from build123d import *

# Parameters (mm, degrees)
SKETCH1_W           = 200
SKETCH1_H           = 180
BOSS_EXTRUDE1_DEPTH = 3
SKETCH2_W           = 200
SKETCH2_H           = 140
BOSS_EXTRUDE2_DEPTH = 5
SKETCH6_W           = 200
SKETCH6_H           = 179.869705491
BOSS_EXTRUDE3_DEPTH = 24
SKETCH7_W           = 155
SKETCH7_H           = 24
CUT_EXTRUDE1_DEPTH  = 179.869705491
SKETCH8_R           = 2
BOSS_EXTRUDE4_DEPTH = 155
SKETCH9_W           = 155
SKETCH9_H           = 5
BOSS_EXTRUDE5_DEPTH = 10
CUT_EXTRUDE3_DEPTH  = 174.869705491
SKETCH12_R          = 7.1
CUT_EXTRUDE4_DEPTH  = 2


with BuildPart() as part:
    # Sketch1 → Boss-Extrude1 (new body)
    with BuildSketch(Plane(origin=(0, 0, 0), x_dir=(1, 0, 0), z_dir=(0, 1, 0))):
        Rectangle(SKETCH1_W, SKETCH1_H)
    extrude(amount=BOSS_EXTRUDE1_DEPTH)

    # Sketch2 → Boss-Extrude2 (add)
    with BuildSketch(Plane.XZ):
        with Locations((0, 20)):
            Rectangle(SKETCH2_W, SKETCH2_H)
    extrude(amount=BOSS_EXTRUDE2_DEPTH)

    # Sketch6 → Boss-Extrude3 (add)
    with BuildSketch(Plane(origin=(0, 3, 0), x_dir=(1, 0, 0), z_dir=(0, 1, 0))):
        with Locations((0, -0.065147254)):
            Rectangle(SKETCH6_W, SKETCH6_H)
    extrude(amount=BOSS_EXTRUDE3_DEPTH)

    # Sketch7 → Cut-Extrude1 (cut)
    with BuildSketch(Plane(origin=(0, 0, -89.869705491), x_dir=(-1, 0, 0), z_dir=(0, 0, -1))):
        with Locations((-17.5, 15)):
            Rectangle(SKETCH7_W, SKETCH7_H)
    extrude(amount=-CUT_EXTRUDE1_DEPTH, mode=Mode.SUBTRACT)

    # Sketch8 → Boss-Extrude4 (add)
    with BuildSketch(Plane.ZY.offset(-95)):
        with Locations(Location((-79.869705491, 13.5, 0), (0, 0, 180))):
            Circle(SKETCH8_R)
    extrude(amount=BOSS_EXTRUDE4_DEPTH)

    # Sketch9 → Boss-Extrude5 (add)
    with BuildSketch(Plane(origin=(0, 3, 0), x_dir=(1, 0, 0), z_dir=(0, 1, 0))):
        with Locations((17.5, -87.5)):
            Rectangle(SKETCH9_W, SKETCH9_H)
    extrude(amount=BOSS_EXTRUDE5_DEPTH)

    # Sketch11 → Cut-Extrude3 (cut)
    with BuildSketch(Plane(origin=(0, 0, -89.869705491), x_dir=(-1, 0, 0), z_dir=(0, 0, -1))):
        Polygon((60, 3), (98, 3), (98, 25), (62, 25), (62, 7), (60, 7), align=None)
    extrude(amount=-CUT_EXTRUDE3_DEPTH, mode=Mode.SUBTRACT)

    # Sketch12 → Cut-Extrude4 (cut)
    with BuildSketch(Plane(origin=(0, 27, 0), x_dir=(1, 0, 0), z_dir=(0, 1, 0))):
        with Locations(Location((-70, -45.032573627, 0), (0, 0, 270))):
            Circle(SKETCH12_R)
        with Locations(Location((-70, -67.516286814, 0), (0, 0, 270))):
            Circle(SKETCH12_R)
        with Locations(Location((-90, -67.516286814, 0), (0, 0, 180))):
            Circle(SKETCH12_R)
        with Locations(Location((-90, -45.032573627, 0), (0, 0, 180))):
            Circle(SKETCH12_R)
    extrude(amount=-CUT_EXTRUDE4_DEPTH, mode=Mode.SUBTRACT)


solid = part.part
Input: part model. Units: mm. Frame: model coordinates. A direction names the side the tool comes from. Give positions to 0.01 mm unless a question says otherwise; leave off trailing zeros. Order: outer loops, then holes, each group sorted by start corner. A loop starts at its lowest first (then second) coordinate and runs counter-clockwise, first axis right, second up. Notation, with made-up numbers: (62.25, 84) - (83.25, 84) arc R25 cw to (83.25, 107) - close; hole circle Ø9 at (-3.75, 50). An arc over 180 degrees is marked (long way). Answer as a JSON object with one key per item and string values. Group by question number.
Q1. First-contact query: pin 1 Ø13 at (x, z) = (-70, 67.52) entering from +Y; pin 2 Ø10 at (x, y) = (67, 13) entering from -Z; pin 3 Ø4 at (x, y) = (-38.5, -2.5) entering from -Z. Flat tips, straight axial feed; report the tip coordinate or a pass-through.
Q2. Cut plane A-A, the plane y = 19. Output: boundary loops of the cut face in (x, z).
Q3. Line query: probe 1 along X at (y, z) = (21, -41.5); probe 2 along Z at (x, y) = (-90, 25.45); probe 3 along Y at (x, z) = (39.5, -46.5). Output: solid intervals per line, ascending.
Q4. Set-up query: faces 5 (the face through (-1, 3, -4)), 6 (the face through (-82.907, 26.014, 67.828)), 7 (the face through (16, 13, 87)). Return all of +Z, -Z, +X, -X, +Y, -Y with unobstructed straight access to the full face (end or side cutting, diameter ignored); none if empty.
Q5. Mould query, pull axis Z, two halves, no side actions, for faces 1 (the face through (-80, 25, -4)), 2 (the face through (-24, 7, 90)), 3 (the face through (-1, -2, -50)), 4 (the face through (-72.7, 26, 51.6)). Classes: pulls with the +Z half, pulls with the -Z half, needs draft (parallel to the pull), parting line crosses it, or undercut.
Q6. Cut plane C-C, the plane x = -70. Output: boundary loops of the cut face in (y, z), then the cut area to 3 significant figures.
Q7. Cut plane B-B, the plane x = 33. Output: boundary loops of the cut face in (y, z), then the cut area to 3 significant figures.
Q8. Cut plane D-D, the plane z = 3.5. Output: boundary loops of the cut face in (x, y).
Results:
{
 "1": {"pin 1": "y = 3", "pin 2": "z = -81.87", "pin 3": "z = -50"},
 "2": {"outline": "(-100, -89.87) - (-98, -89.87) - (-98, 85) - (-62, 85) - (-62, -89.87) - (-60, -89.87) - (-60, 90) - (-100, 90) - close; (95, -89.87) - (100, -89.87) - (100, 90) - (95, 90) - close"},
 "3": {"probe 1": "-100 to -98, -62 to -60, 95 to 100", "probe 2": "-89.87 to 37.93, 52.13 to 60.42, 74.62 to 90", "probe 3": "-5 to 3"},
 "4": {"face 5": "-Z", "face 6": "+Y", "face 7": "+Z, +Y"},
 "5": {"face 1": "needs draft", "face 2": "pulls with the +Z half", "face 3": "pulls with the -Z half", "face 4": "undercut"},
 "6": {"outline": "(-5, -50) - (0, -50) - (0, -90) - (3, -90) - (3, 85) - (25, 85) - (25, 74.62) - (27, 74.62) - (27, 90) - (-5, 90) - close; (25, -89.87) - (27, -89.87) - (27, 37.93) - (25, 37.93) - close; (25, 52.13) - (27, 52.13) - (27, 60.42) - (25, 60.42) - close", "area": "1,650 mm^2"},
 "7": {"outline": "(-5, -50) - (0, -50) - (0, -90) - (3, -90) - (3, 85) - (13, 85) - (13, 90) - (-5, 90) - close; circle Ø4 at (13.5, -79.87)", "area": "1,300 mm^2"},
 "8": {"outline": "(-100, -5) - (100, -5) - (100, 27) - (95, 27) - (95, 3) - (-98, 3) - (-98, 25) - (-62, 25) - (-62, 7) - (-60, 7) - (-60, 27) - (-100, 27) - close"}
}
